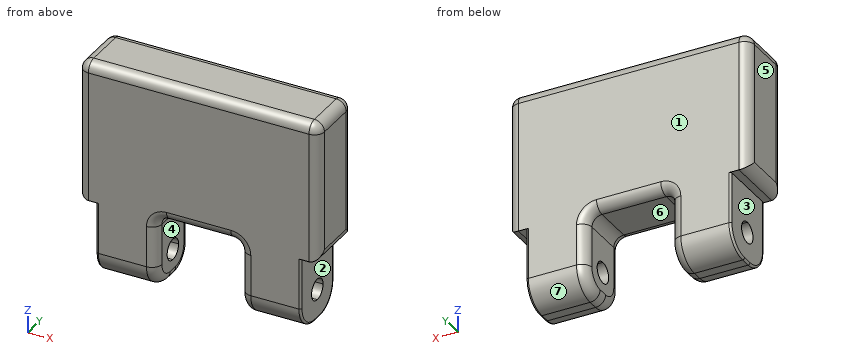
from build123d import *

# Parameters (mm, degrees)
F0_W     = 3
F0_H     = 3.8
F1_DEPTH = 3
F3_DEPTH = 11.101
F4_R     = 1.25
F5_F1_R  = 0.5
F5_F2_R  = 0.5
F6_R     = 0.1


with BuildPart() as f1:
    # F0 (on Front) → F1 (new body)
    with BuildSketch(Plane.XZ):
        Polygon((6, -3.5), (6, 3.5), (0, 3.5), (0, -3.5), (2.1, -3.5), (5.1, -3.5), align=None)
        with Locations((3.6, -5.4)):
            Rectangle(F0_W, F0_H)
        with Locations((-3.6, -5.4)):
            Rectangle(F0_W, F0_H)
        Polygon((0, -3.5), (0, 3.5), (-6, 3.5), (-6, -3.5), (-5.1, -3.5), (-2.1, -3.5), align=None)
    extrude(amount=F1_DEPTH)

    # F2 (on face) → F3 (cut, through all)
    with BuildSketch(Plane.YZ.offset(5.1)):
        with BuildLine():
            ThreePointArc((-1.5, -5.275), (-2.025, -5.8), (-1.5, -6.325))
            Line((-1.5, -6.325), (-1.5, -5.275))
        make_face()
        with BuildLine():
            Line((-1.5, -5.275), (-1.5, -6.325))
            ThreePointArc((-1.5, -6.325), (-1.1287689399, -6.1712310601), (-0.975, -5.8))
            ThreePointArc((-0.975, -5.8), (-1.1287689399, -5.4287689399), (-1.5, -5.275))
        make_face()
    extrude(amount=-F3_DEPTH, mode=Mode.SUBTRACT)

    # F4
    f4_edges = [f1.edges().sort_by_distance(p)[0] for p in [
        (-3.6, -3, -7.3),
        (-3.6, 0, -7.3),
        (3.6, -3, -7.3),
        (3.6, 0, -7.3),
    ]]
    fillet(f4_edges, radius=F4_R)

    # F5: fillet of radius 0.5 on 14 edges, made by hand

    # F5_f1
    f5_f1_edges = [f1.edges().sort_by_distance(p)[0] for p in [
        (-2.1, -1.5, -3.5),
        (2.1, -1.5, -3.5),
    ]]
    fillet(f5_f1_edges, radius=F5_F1_R)

    # F5_f2
    f5_f2_edges = [f1.edges().sort_by_distance(p)[0] for p in [
        (0, 0, -3.5),
        (0, -3, -3.5),
        (-6, -1.5, 3.5),
        (-6, -1.5, -3.5),
        (-6, 0, 0),
        (-6, -3, 0),
        (6, -1.5, -3.5),
        (6, -1.5, 3.5),
        (6, 0, 0),
        (6, -3, 0),
        (0, 0, 3.5),
        (0, -3, 3.5),
        (-1.9535533906, -3, -3.6464466094),
        (1.9535533906, -3, -3.6464466094),
        (-1.9535533906, 0, -3.6464466094),
        (1.9535533906, 0, -3.6464466094),
    ]]
    fillet(f5_f2_edges, radius=F5_F2_R)

    # F6
    f6_edges = [f1.edges().sort_by_distance(p)[0] for p in [
        (-5.1, -2.633883, -6.933883),
        (5.1, -3, -4.775),
    ]]
    fillet(f6_edges, radius=F6_R)


solid = f1.part
Verification items for the finished model (mm, model axes). Face numbers are marked on the shaded views. A direction names the side the tool comes from. Coordinates: 2 decimals unless noted, no trailing zeros. Write each loop counter-clockwise with the first axis right and the second up, starting at its lowest first coordinate (ties: lowest second). Pieces come first, ordered by that corner, then holes. Notation, with made-up numbers: M -31,0.25 L -12,0.25 A31 ccw -12,31.25 Z; hole C 77.5,59 d11. An arc over 180 degrees is marked long. One line per question, with ' | ' between items.
1) Material ranges on L1, parallel to X at y = -1.05, z = -6.25; L2, parallel to Z at x = -0.5, y = -0.8; L3, parallel to Y at x = 3.25, z = -6, recorded low to high.
Solutions:
L1: -5.1 to -2.1, 2.1 to 5.1 | L2: -3.5 to 3.5 | L3: -3 to -1.99, -1.01 to 0
2) Sectioned sample at C-C on x = 0.5. Record the cut outline in (y, z), then the cut area to 3 significant figures.
Solutions:
outline: M -3,-3 A0.5 ccw -2.5,-3.5 L -0.5,-3.5 A0.5 ccw 0,-3 L 0,3 A0.5 ccw -0.5,3.5 L -2.5,3.5 A0.5 ccw -3,3 Z | area: 20.8 mm^2
3) Access from +Z, -Z, +X, -X, +Y, -Y to the whole of each face (thin tool, end or side, straight path). Record for the marked faces 1, 2, 3 and 4.
Solutions:
face 1: +Z, -Z, +X, -X, +Y | face 2: -Z, +X, +Y, -Y | face 3: -Z, -X, +Y, -Y | face 4: -Z, +Y, -Y
4) Depth check by flat-ended pin: pin 1 Ø1.4 at (y, z) = (-1, -5) entering from -X. Enter the tip coordinate at first touch or a pass-through.
Solutions:
pin 1: x = -5.1
5) Sectioned sample at B-B on z = -4.5. Record the cut outline in (x, y).
Solutions:
outline: M -5.1,-2.9 A0.1 ccw -5,-3 L -2.6,-3 A0.5 ccw -2.1,-2.5 L -2.1,-0.5 A0.5 ccw -2.6,0 L -5,0 A0.1 ccw -5.1,-0.1 Z; M 2.1,-2.5 A0.5 ccw 2.6,-3 L 5,-3 A0.1 ccw 5.1,-2.9 L 5.1,-0.1 A0.1 ccw 5,0 L 2.6,0 A0.5 ccw 2.1,-0.5 Z
6) Release check for a two-part mould opening along X. For the marked faces 5, 6 and 7 record: +X half, -X half, draft (parallel to the pull), parting line (faces both ways), or undercut.
Solutions:
face 5: -X half | face 6: undercut | face 7: draft
7) Sectioned sample at A-A on x = 3.75. Record the cut outline in (y, z) (3 decimals).
Solutions:
outline: M -3,-6.05 A1.25 ccw -1.75,-7.3 L -1.25,-7.3 A1.25 ccw 0,-6.05 L 0,3 A0.5 ccw -0.5,3.5 L -2.5,3.5 A0.5 ccw -3,3 Z; hole C -1.5,-5.8 d1.05
